Part model, mm, in its own coordinate system. A direction names the side the tool comes from. Round coordinates to 2 decimals unless told otherwise and drop trailing zeros. Loops run counter-clockwise (first coordinate to the right, second up) from the corner with the lowest first, then second, coordinate; pieces in that order, holes last. Notation, with made-up numbers: M -19,64 L 13,64 A19 ccw 13,96 Z; hole C 59,20 d2. An arc over 180 degrees is marked long. Answer as CSV lines item,"result". Start each with the question number.
Item 1: Wall check: line 1 (X direction, y = -12, z = 0); line 2 (X direction, y = -2.5, z = 0) (3 decimals); line 3 (Z direction, x = 4.5, y = 6.5). Give the ranges that are in metal, low to high.
Item 2: Mould opens along Z. For faces 4 (the flat face through (-3.3, -20.5, 0.1)), 5 (the flat face through (-0.27, 3.944, -2.235)) say: pulls with the +Z half, pulls with the -Z half, needs draft (parallel to the pull), parting line crosses it, or undercut.
Item 3: Which spindle directions (+Z, -Z, +X, -X, +Y, -Y) get a long thin tool onto all of the face, cutting with end or side? Do faces 1 (the flat face through (-2.2, 8, -1.2)), 2 (the flat face through (0, -6, 0)), 3 (the flat face through (0, -7.5, 0)). Say none if no direction does.
Item 4: Band-saw the part on D-D (y = -8.5). Give the cut face in (x, z), and give its area (3 significant figures).
Item 5: Band-saw the part on A-A (y = 4.25). Give the cut face in (x, z), and give its area (3 significant figures).
Item 6: Band-saw the part on C-C (x = 0). Give the cut face in (y, z) (3 decimals), and give its area (3 significant figures).
Item 7: Drop flat-ended pins along their axis: pin 1 Ø4 at (y, z) = (-5, 0.5) entering from -X; pin 2 Ø2.5 at (x, z) = (0, 0) entering from +Y; pin 3 Ø3.5 at (x, z) = (0, 0) entering from -Y. Give the stop position or say it passes through.
Item 8: Band-saw the part on B-B (z = 0). Give the cut face in (x, y) (3 decimals).
```python
from build123d import *

# Parameters (mm, degrees)
SKETCH1_R           = 5
BOSS_EXTRUDE1_DEPTH = 8
BOSS_EXTRUDE2_START = 6
SKETCH2_R           = 5
SKETCH2_R_2         = 2.175
BOSS_EXTRUDE2_DEPTH = 6
BOSS_EXTRUDE3_START = 1.5
SKETCH3_R           = 5
BOSS_EXTRUDE3_DEPTH = 1.5
BOSS_EXTRUDE4_START = 13
SKETCH4_R           = 5
BOSS_EXTRUDE4_DEPTH = 13


with BuildPart() as part:
    # Sketch1 → Boss-Extrude1 (new body)
    with BuildSketch(Plane(origin=(0, 0, 0), x_dir=(1, 0, 0), z_dir=(0, 1, 0))):
        with Locations(Location((0, 0, 0), (0, 0, 270))):
            Circle(SKETCH1_R)
        Polygon((1.577657476, -2.066639032), (2.57859064, 0.332971936), (1.000933165, 2.399610968), (-1.577657476, 2.066639032), (-2.57859064, -0.332971936), (-1.000933165, -2.399610968), align=None, mode=Mode.SUBTRACT)
    extrude(amount=BOSS_EXTRUDE1_DEPTH)

    # Sketch2 → Boss-Extrude2 (add)
    with BuildSketch(Plane.XZ.offset(BOSS_EXTRUDE2_START)):
        with Locations(Location((0, 0, 0), (0, 0, 270))):
            Circle(SKETCH2_R)
        with Locations(Location((0, 0, 0), (0, 0, 270))):
            Circle(SKETCH2_R_2, mode=Mode.SUBTRACT)
    extrude(amount=-BOSS_EXTRUDE2_DEPTH)

    # Sketch3 → Boss-Extrude3 (add)
    with BuildSketch(Plane.XZ.offset(6).offset(BOSS_EXTRUDE3_START)):
        with Locations(Location((0, 0, 0), (0, 0, 270))):
            Circle(SKETCH3_R)
    extrude(amount=-BOSS_EXTRUDE3_DEPTH)

    # Sketch4 → Boss-Extrude4 (add)
    with BuildSketch(Plane.XZ.offset(7.5).offset(BOSS_EXTRUDE4_START)):
        with Locations(Location((0, 0, 0), (0, 0, 270))):
            Circle(SKETCH4_R)
        with BuildLine():
            Line((-1.747140521, 2.5), (1.747140521, 2.5))
            ThreePointArc((1.747140521, 2.5), (0, -3.05), (-1.747140521, 2.5))
        make_face(mode=Mode.SUBTRACT)
    extrude(amount=-BOSS_EXTRUDE4_DEPTH)


solid = part.part
```
Answer block:
1,line 1,"x = -5 to -3.05, 3.05 to 5"
1,line 2,"x = -5 to -2.175, 2.175 to 5"
1,line 3,"z = -2.18 to 2.18"
2,face 4,"needs draft"
2,face 5,"undercut"
3,face 1,"+Z, -Z, +X, -X, +Y"
3,face 2,"+Y"
3,face 3,"-Y"
4,outline,"C 0,0 d10; hole M -1.75,2.5 A3.05 ccw long 1.75,2.5 Z"
4,area,"50.6 mm^2"
5,outline,"C 0,0 d10; hole M -2.58,0.33 L -1.58,-2.07 L 1,-2.4 L 2.58,-0.33 L 1.58,2.07 L -1,2.4 Z"
5,area,"61.0 mm^2"
6,outline,"M -20.5,-5 L 8,-5 L 8,-2.27 L 0,-2.27 L 0,-2.175 L -6,-2.175 L -6,2.175 L 0,2.175 L 0,2.27 L 8,2.27 L 8,5 L -20.5,5 L -20.5,2.5 L -7.5,2.5 L -7.5,-3.05 L -20.5,-3.05 Z"
6,area,"150 mm^2"
7,pin 1,"stops at x = -5"
7,pin 2,"stops at y = -6"
7,pin 3,"stops at y = -7.5"
8,outline,"M -5,-20.5 L -3.05,-20.5 L -3.05,-7.5 L 3.05,-7.5 L 3.05,-20.5 L 5,-20.5 L 5,8 L 2.44,8 L 2.44,0 L 2.175,0 L 2.175,-6 L -2.175,-6 L -2.175,0 L -2.44,0 L -2.44,8 L -5,8 Z"
